Input: part model. Units: mm. Frame: model coordinates. Face numbers are marked on the shaded views. A direction names the side the tool comes from. Coordinates: 2 decimals unless noted, no trailing zeros. Loops run counter-clockwise (first coordinate to the right, second up) from the corner with the lowest first, then second, coordinate; pieces in that order, holes last. Notation, with made-up numbers: M 61,61 L 78,61 A19 ccw 78,89 Z; hole C -34.5,13.5 d11. An arc over 180 degrees is marked long. Use a Markdown table: item, result. Add a question column.
1. Section D-D on y = -27.5. Output: boundary loops of the cut face in (x, z).
2. Section B-B on x = 5.75. Output: boundary loops of the cut face in (y, z).
3. Pin query (flat end, axial travel): pin 1 (3 mm diameter, centred on x = 3, y = -17.5, fed in from +Z); pin 2 (2 mm diameter, centred on x = 3, y = 3.5, fed in from +Z); pin 3 (3 mm diameter, centred on x = 1.5, y = -4, fed in from -Z). Return the tip coordinate at first contact, or that it passes through.
4. Draft query along Y for the marked faces 1, 2 and 3. Return one class per face: +Y half, -Y half, draft (parallel to the pull), parting line (faces both ways), or undercut.
5. Line query: L1, parallel to X at y = -32.15, z = 16.5; L2, parallel to Z at x = 5.25, y = -15.5; L3, parallel to Y at x = 1.5, z = 16.5. Output: solid intervals per line, ascending. Write a range as [from, to].
6. Section A-A on z = 0. Output: boundary loops of the cut face in (x, y).
7. Section C-C on y = 1. Output: boundary loops of the cut face in (x, z).
8. Set-up query: the marked faces 4, 5 and 6. Return all of +Z, -Z, +X, -X, +Y, -Y with unobstructed straight access to the full face (end or side cutting, diameter ignored); none if empty.
```python
from build123d import *

# Parameters (mm, degrees)
EXTRUDE_1_DEPTH     = 8
CUT_EXTRUDE_1_DEPTH = 19.248287591
SKETCH_4_W          = 8
SKETCH_4_H          = 26
EXTRUDE_2_DEPTH     = 24.15
SKETCH_5_W          = 8
SKETCH_5_H          = 39.090909091
SKETCH_5_R          = 2.25
EXTRUDE_3_DEPTH     = 5


with BuildPart() as part:
    # Эскиз1 → Бобышка-Вытянуть1 (new body)
    with BuildSketch(Plane(origin=(0, 0, 0), x_dir=(0, 0, -1), z_dir=(1, 0, 0))):
        with BuildLine():
            Line((-13, -5), (-13, -10))
            Line((-13, -10), (13, -10))
            Line((13, -10), (13, -5))
            ThreePointArc((13, -5), (9.464466094, -3.535533906), (8, 0))
            ThreePointArc((8, 0), (0, 8), (-8, 0))
            ThreePointArc((-8, 0), (-9.464466094, -3.535533906), (-13, -5))
        make_face()
    extrude(amount=EXTRUDE_1_DEPTH)

    # Эскиз2 → Вырез-Вытянуть1 (cut, through all)
    with BuildSketch(Plane(origin=(8, 0, 0), x_dir=(0, 0, -1), z_dir=(1, 0, 0))):
        Polygon((5.773502692, 0), (2.886751346, 5), (-2.886751346, 5), (-5.773502692, 0), (-2.886751346, -5), (2.886751346, -5), align=None)
    extrude(amount=-CUT_EXTRUDE_1_DEPTH, mode=Mode.SUBTRACT)

    # Эскиз4 → Бобышка-Вытянуть2 (add)
    with BuildSketch(Plane.XZ.offset(10)):
        with Locations((4, 0)):
            Rectangle(SKETCH_4_W, SKETCH_4_H)
    extrude(amount=EXTRUDE_2_DEPTH)

    # Эскиз5 → Бобышка-Вытянуть3 (add)
    with BuildSketch(Plane.XZ.offset(34.15)):
        with Locations((4, -1e-09)):
            Rectangle(SKETCH_5_W, SKETCH_5_H)
        with Locations(Location((4, -16.5, 0), (0, 0, 270))):
            Circle(SKETCH_5_R, mode=Mode.SUBTRACT)
        with Locations(Location((4, 16.5, 0), (0, 0, 270))):
            Circle(SKETCH_5_R, mode=Mode.SUBTRACT)
    extrude(amount=-EXTRUDE_3_DEPTH)


solid = part.part
```
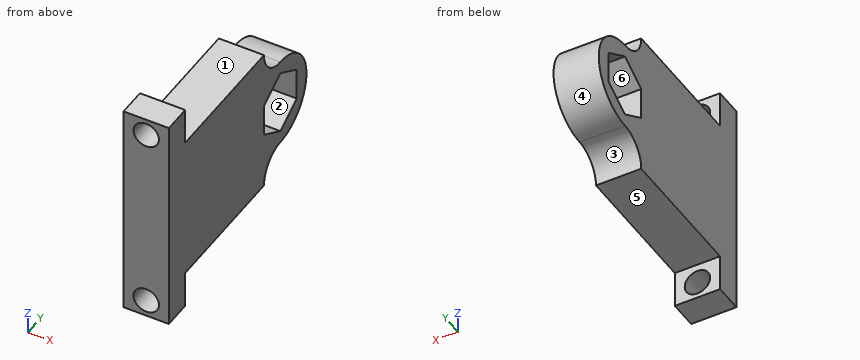
Answers below:
| question | item | result |
|---|---|---|
| 1 | outline | M 0,-13 L 8,-13 L 8,13 L 0,13 Z |
| 2 | outline | M -34.15,-19.55 L -29.15,-19.55 L -29.15,-17.91 L -34.15,-17.91 Z; M -34.15,-15.09 L -29.15,-15.09 L -29.15,-13 L -5,-13 A5 cw 0,-8 A8 ccw 0,8 A5 cw -5,13 L -29.15,13 L -29.15,15.09 L -34.15,15.09 Z; M -34.15,17.91 L -29.15,17.91 L -29.15,19.55 L -34.15,19.55 Z; hole M -5,-2.89 L 0,-5.77 L 5,-2.89 L 5,2.89 L 0,5.77 L -5,2.89 Z |
| 3 | pin 1 | stops at z = 13 |
| 3 | pin 2 | stops at z = 7.6 |
| 3 | pin 3 | stops at z = -13 |
| 4 | face 1 | draft |
| 4 | face 2 | undercut |
| 4 | face 3 | +Y half |
| 5 | L1 | x = [0, 1.75], [6.25, 8] |
| 5 | L2 | z = [-13, 13] |
| 5 | L3 | y = [-34.15, -29.15] |
| 6 | outline | M 0,-34.15 L 8,-34.15 L 8,-5 L 0,-5 Z; M 0,5 L 8,5 L 8,8 L 0,8 Z |
| 7 | outline | M 0,-7.94 L 8,-7.94 L 8,-5.2 L 0,-5.2 Z; M 0,5.2 L 8,5.2 L 8,7.94 L 0,7.94 Z |
| 8 | face 4 | +X, -X, +Y |
| 8 | face 5 | -Z, +X, -X, +Y |
| 8 | face 6 | +X, -X |
